```python
from build123d import *
from build123d.topology import SkipClean

# Parameters (mm, degrees)
SKETCH1_R           = 2
BOSS_EXTRUDE1_DEPTH = 15
SKETCH3_R           = 3
BOSS_EXTRUDE2_DEPTH = 1
FILLET3_R           = 1


with BuildPart() as part:
    # Sketch1 → Boss-Extrude1 (new body)
    with BuildSketch(Plane(origin=(0, 0, 0), x_dir=(1, 0, 0), z_dir=(0, 1, 0))):
        with Locations(Location((0, 0, 0), (0, 0, 270))):
            Circle(SKETCH1_R)
    extrude(amount=BOSS_EXTRUDE1_DEPTH)

    # Sketch2 → Revolve1 (revolve)
    with SkipClean():  # the faces are left unmerged after this step: merging them gives an invalid solid
        with BuildSketch(Plane.XY):
            with BuildLine():
                Line((2, 15), (-2, 15))
                ThreePointArc((-2, 15), (0, 17), (2, 15))
            make_face()
        revolve(axis=Axis((2, 15, 0), (-1, 0, 0)))

    # Sketch3 → Boss-Extrude2 (add)
    with BuildSketch(Plane.XZ):
        with Locations(Location((0, 0, 0), (0, 0, 270))):
            Circle(SKETCH3_R)
    extrude(amount=BOSS_EXTRUDE2_DEPTH)

    # Fillet3
    fillet3_edges = [part.edges().sort_by_distance(p)[0] for p in [
        (0, 0, -2),
    ]]
    fillet(fillet3_edges, radius=FILLET3_R - 0.0001)  # a hair under: the kernel refuses the full size


solid = part.part
```
The model under review builds one solid part; all positions refer to its coordinate system, in mm. A direction names the side the tool comes from. Give positions to 0.01 mm unless a question says otherwise; leave off trailing zeros. Loops run counter-clockwise (first coordinate to the right, second up) from the corner with the lowest first, then second, coordinate; pieces in that order, holes last. Notation, with made-up numbers: (54, 49.5) - (109, 49.5) arc R18 cw to (109, 71.5) - close; hole circle Ø10 at (10, -27.75). An arc over 180 degrees is marked (long way). Answer as a JSON object with one key per item and string values.
Q1. Add section B-B on y = 6. State the section outline as (x, z) points, plus the area to 3 significant figures.
Worked out:
{"outline": "circle Ø4 at (0, 0)", "area": "12.6 mm^2"}
Q2. For faces 1 (the cylindrical face through (0.9, -0.49, -2.86)), 2 (the cylindrical face through (-2, 8, 0)), list the 3-axis set-ups (+Z, -Z, +X, -X, +Y, -Y) from which the entire face can be reached by the end or side of a thin tool; tool diameter is ignored.
Worked out:
{"face 1": "+Y, -Y", "face 2": "+Y"}
Q3. Insertion check: pin 1 (1 mm diameter, centred on y = 2.5, z = 1.5, fed in from +X); pin 2 (3 mm diameter, centred on y = 11.5, z = 1.5, fed in from -X); pin 3 (3 mm diameter, centred on x = -1.5, z = -1.5, fed in from +Y). Each pin has a flat end and moves straight along its axis. Give the tip position at first contact, or say it passes through.
Worked out:
{"pin 1": "stops at x = 1.73", "pin 2": "stops at x = -2", "pin 3": "stops at y = 16.9"}
Q4. To check wall thickness, follow line 1 along Z through (x, y) = (0.1, 2.5); line 2 along X through (y, z) = (12.25, -0.55); line 3 along Z through (x, y) = (-0.85, 2.75). State the ranges of each line that lie inside material, in increasing order.
Worked out:
{"line 1": "z = -2 to 2", "line 2": "x = -1.92 to 1.92", "line 3": "z = -1.81 to 1.81"}
